```python
from build123d import *

# Parameters (mm, degrees)
F0_R     = 8
F1_DEPTH = 10
F2_R     = 5
F3_DEPTH = 20
F4_SIZE  = 1
F6_DEPTH = 5


with BuildPart() as f1:
    # F0 (on Front) → F1 (new body)
    with BuildSketch(Plane.XZ):
        Circle(F0_R)
    extrude(amount=F1_DEPTH)

    # F2 (on face) → F3 (join)
    with BuildSketch(Plane.XZ.offset(10)):
        Circle(F2_R)
    extrude(amount=F3_DEPTH)

    # F4
    f4_edges = [f1.edges().sort_by_distance(p)[0] for p in [
        (-5, -30, 0),
        (-8, 0, 0),
    ]]
    chamfer(f4_edges, length=F4_SIZE)

    # F5 (on face) → F6 (cut)
    with BuildSketch(Plane(origin=(0, 0, 0), x_dir=(-1, 0, 0), z_dir=(0, 1, 0))):
        Polygon((-4.618402, 0.06081), (-2.361864, -3.969249), (2.256538, -4.030058), (4.618402, -0.06081), (2.361864, 3.969249), (-2.256538, 4.030058), align=None)
    extrude(amount=-F6_DEPTH, mode=Mode.SUBTRACT)


solid = f1.part
```
Can you work these out from the model? Positions are in its coordinate system, mm. A direction names the side the tool comes from. Give positions to 0.01 mm unless a question says otherwise; leave off trailing zeros. Loops run counter-clockwise (first coordinate to the right, second up) from the corner with the lowest first, then second, coordinate; pieces in that order, holes last. Notation, with made-up numbers: M -6,45.25 L 29,45.25 A25 cw 29,77.25 Z; hole C 70.5,-11.5 d6. An arc over 180 degrees is marked long. Use CSV: the item, a comma, the result in double quotes. Start each with the question number.
1. If I drill on L1, parallel to Y at x = -3.5, z = -5.75; L2, parallel to Z at x = -1.5, y = -2.25; L3, parallel to Y at x = -3.25, z = 2, over which ranges is the centre line in solid material (lowest first)?
2. On a 3-axis mill with a long thin cutter (end or side, diameter ignored), from which of +Z, -Z, +X, -X, +Y, -Y can I reach the whole of each face in a straight line? I mean faces 4 (the face through (0, -30, 0)), 5 (the face through (5.2, -10, 0.1)), 6 (the face through (3.506, -2.465, -1.926)). Say none if no direction works.
3. Imagine slicing it at B-B, the plane x = 0. Write out the boundary of the cut face in (y, z).
4. Imagine slicing it at A-A, the plane y = -2.5. Write out the boundary of the cut face in (x, z), plus the area to 3 significant figures.
5. If we mould it in two halves opening along X, with no side actions, what happens to faces 1 (the face through (-1.08, -19.37, -4.88)), 2 (the face through (-3.2, 0, -3)), 3 (the face through (3.421, -2.465, 2.073))? For each: released by +X, released by -X, zero draft, split by the parting line, or undercut.
6. Imagine slicing it at D-D, the plane y = -7. Write out the boundary of the cut face in (x, z).
7. Imagine slicing it at C-C, the plane y = -13. Write out the boundary of the cut face in (x, z).
8. For P1, Ø1, axis at y = -22, z = 6, coming from the -X side; P2, Ø8, axis at y = -16, z = -3.5, coming from the -X side; P3, Ø1, axis at y = -22.5, z = 1, coming from the +X side; P4, Ø5, axis at x = 3.5, y = -20.5, coming from the -Z side, each with a flat end and sliding along its axis, tell me the tip position at first contact or that it passes through.
Response values:
1,L1,"-10 to 0"
1,L2,"-7.86 to -4.02, 3.98 to 7.86"
1,L3,"-30 to -5"
2,face 4,"+Z, -Z, +X, -X, -Y"
2,face 5,"-Y"
2,face 6,"+Y"
3,outline,"M -30,-4 L -29,-5 L -10,-5 L -10,-8 L -1,-8 L 0,-7 L 0,-4 L -5,-4 L -5,4 L 0,4 L 0,7 L -1,8 L -10,8 L -10,5 L -29,5 L -30,4 Z"
4,outline,"C 0,0 d16; hole M -4.62,-0.06 L -2.26,-4.03 L 2.36,-3.97 L 4.62,0.06 L 2.26,4.03 L -2.36,3.97 Z"
4,area,"146 mm^2"
5,face 1,"split by the parting line"
5,face 2,"zero draft"
5,face 3,"undercut"
6,outline,"C 0,0 d16"
7,outline,"C 0,0 d10"
8,P1,"through"
8,P2,"x = -5"
8,P3,"x = 4.97"
8,P4,"z = -4.9"
